Input: part model. Units: mm. Frame: model coordinates. Face numbers are marked on the shaded views. A direction names the side the tool comes from. Give positions to 0.01 mm unless a question says otherwise; leave off trailing zeros. Loops run counter-clockwise (first coordinate to the right, second up) from the corner with the lowest first, then second, coordinate; pieces in that order, holes last. Notation, with made-up numbers: (-26.75, -9) - (-17.75, -9) arc R21 ccw to (-17.75, -1) - close; hole circle Ø6 at (74, 63). An arc over 180 degrees is marked (long way). Answer as a JSON object with one key per item and string values.
from build123d import *

# Parameters (mm, degrees)
F0_W     = 40
F0_H     = 40
F1_DEPTH = 30
F2_R     = 5
F3_T     = -2.5
F4_W     = 20.2598124743
F4_H     = 19.6875007823
F5_DEPTH = 61


# Not quite as in the source:
# - a shell that OpenCascade refuses in one call is made with other operations: the cavity is built on its own and cut out


with BuildPart() as f1:
    # F0 (on Top) → F1 (new body)
    with BuildSketch(Plane.XY):
        Rectangle(F0_W, F0_H)
    extrude(amount=F1_DEPTH)

    # F2
    f2_edges = [f1.edges().sort_by_distance(p)[0] for p in [
        (-20, -20, 15),
        (20, -20, 15),
        (0, -20, 0),
        (0, -20, 30),
        (-20, 0, 30),
        (20, 0, 30),
        (0, 20, 30),
        (20, 20, 15),
        (20, 0, 0),
        (-20, 20, 15),
        (-20, 0, 0),
    ]]
    fillet(f2_edges, radius=F2_R)

    # F3: a shell. OpenCascade refuses it in one call, so the cavity is built on its own and cut out:
    # the body offset inwards by the wall thickness, plus a prism from it out through each open face.
    f3_core = offset(f1.part, amount=F3_T, mode=Mode.PRIVATE)
    f3_exits = [f3_core.faces().sort_by_distance(p)[0] for p in [
        (0, 0, 27.5),
    ]]
    add(f3_core, mode=Mode.SUBTRACT)
    extrude(f3_exits, amount=-F3_T, mode=Mode.SUBTRACT)

    # F4 (on Front) → F5 (cut)
    with BuildSketch(Plane.XZ):
        with Locations((10.1299062371, 14.9945500307)):
            Rectangle(F4_W, F4_H)
    extrude(amount=F5_DEPTH, mode=Mode.SUBTRACT)


solid = f1.part
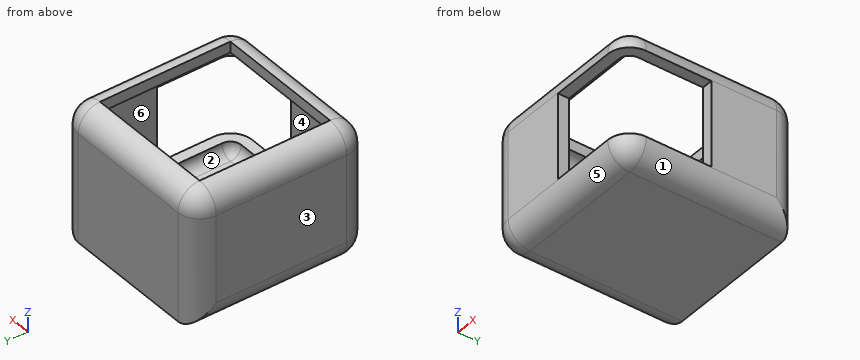
Item 1: Cut plane A-A (y = -14). Return loops of the section in (x, z), then the cut area to 3 significant figures.
Geometry check:
{"outline": "(-20, 5) arc R5 ccw to (-15, 0) - (15, 0) arc R5 ccw to (20, 5) - (20, 5.15) - (17.5, 5.15) - (17.5, 5) arc R2.5 cw to (15, 2.5) - (-15, 2.5) arc R2.5 cw to (-17.5, 5) - (-17.5, 25) arc R2.5 cw to (-15, 27.5) - (-15, 30) arc R5 ccw to (-20, 25) - close; (15, 27.5) arc R2.5 cw to (17.5, 25) - (17.5, 24.84) - (20, 24.84) - (20, 25) arc R5 ccw to (15, 30) - close", "area": "185 mm2"}
Item 2: Cut plane B-B (x = 9.5). Return loops of the section in (y, z), then the cut area to 3 significant figures.
Geometry check:
{"outline": "(-20, 5) arc R5 ccw to (-15, 0) - (20, 0) - (20, 25) arc R5 ccw to (15, 30) - (15, 27.5) arc R2.5 cw to (17.5, 25) - (17.5, 2.5) - (-15, 2.5) arc R2.5 cw to (-17.5, 5) - (-17.5, 5.15) - (-20, 5.15) - close; (-20, 24.84) - (-17.5, 24.84) - (-17.5, 25) arc R2.5 cw to (-15, 27.5) - (-15, 30) arc R5 ccw to (-20, 25) - close", "area": "189 mm2"}
Item 3: Access query for the marked faces 1 and 2. Directions: +Z, -Z, +X, -X, +Y, -Y. A direction counts if a zero-diameter tool reaches every point of the face in a straight line with its end or side. Return the directions, or none.
Geometry check:
{"face 1": "-Z, +X, +Y, -Y", "face 2": "none"}
Item 4: Material intervals for line 1 (X direction, y = 12.5, z = 23.5); line 2 (Y direction, x = -7.5, z = 4.75); line 3 (X direction, y = -11, z = 10.5), sorted ascending. Write a range as [from, to].
Geometry check:
{"line 1": "x = [-20, -17.5], [17.5, 20]", "line 2": "y = [-19.99, -17.49], [17.5, 20]", "line 3": "x = [-20, -17.5]"}
Item 5: Cut plane D-D (y = 11). Return loops of the section in (x, z), then the cut area to 3 significant figures.
Geometry check:
{"outline": "(-20, 5) arc R5 ccw to (-15, 0) - (15, 0) arc R5 ccw to (20, 5) - (20, 25) arc R5 ccw to (15, 30) - (15, 27.5) arc R2.5 cw to (17.5, 25) - (17.5, 5) arc R2.5 cw to (15, 2.5) - (-15, 2.5) arc R2.5 cw to (-17.5, 5) - (-17.5, 25) arc R2.5 cw to (-15, 27.5) - (-15, 30) arc R5 ccw to (-20, 25) - close", "area": "234 mm2"}
Item 6: Mould query, pull axis Z, two halves, no side actions, for the marked faces 3, 4, 5 and 6. Classes: released by +Z, released by -Z, zero draft, split by the parting line, or undercut.
Geometry check:
{"face 3": "zero draft", "face 4": "undercut", "face 5": "released by -Z", "face 6": "undercut"}
Item 7: Contact query for flat-ended pins moving along their axis: P1, Ø2, axis at y = -19, z = 16.5, coming from the +X side; P2, Ø24, axis at x = -0.5, y = 0, coming from the +Z side; P3, Ø0.8, axis at x = 0.5, z = 29, coming from the +Y side. Output: stop coordinate, or through.
Geometry check:
{"P1": "stops at x = 0", "P2": "stops at z = 2.5", "P3": "stops at y = 18.47"}
Item 8: Cut plane C-C (z = 8.5). Return loops of the section in (x, y).
Geometry check:
{"outline": "(-20, -15) arc R5 ccw to (-15, -20) - (0, -20) - (0, -17.5) - (-15, -17.5) arc R2.5 cw to (-17.5, -15) - (-17.5, 15) arc R2.5 cw to (-15, 17.5) - (15, 17.5) arc R2.5 cw to (17.5, 15) - (17.5, 0) - (20, 0) - (20, 15) arc R5 ccw to (15, 20) - (-15, 20) arc R5 ccw to (-20, 15) - close"}
